CAD build for the part. Positions are in the model's coordinates, mm. A direction names the side the tool comes from. Give positions to 0.01 mm unless a question says otherwise; leave off trailing zeros. Write each loop counter-clockwise with the first axis right and the second up, starting at its lowest first coordinate (ties: lowest second). Pieces come first, ordered by that corner, then holes. Notation, with made-up numbers: (1, 19) - (13, 19) arc R30 cw to (13, 53) - close; hole circle Ø10 at (66.25, 86). An arc over 180 degrees is marked (long way). Answer as a JSON object with one key per item and string values.
from build123d import *

# Parameters (mm, degrees)
SKETCH_1_R          = 2.1
EXTRUDE_1_DEPTH     = 2
CUT_EXTRUDE_1_DEPTH = 94.621578709
CHAMFER_1_SIZE      = 2
SKETCH_4_R          = 1
CUT_EXTRUDE_2_DEPTH = 94.621578709
CHAMFER_2_SIZE      = 4
SKETCH_7_R          = 1.6
CUT_EXTRUDE_3_DEPTH = 94.621578709


with BuildPart() as part:
    # 草图1 → 凸台-拉伸1 (new, symmetric)
    with BuildSketch(Plane.XY):
        with BuildLine():
            Line((11, 0), (-11, 0))
            Line((-11, 0), (-11, -82))
            Line((-11, -82), (-31, -82))
            Line((-31, -82), (-31, 20))
            Line((-31, 20), (45, 20))
            Line((45, 20), (45, -33.306562209))
            ThreePointArc((45, -33.306562209), (42.507569164, -36.65839818), (38.580111783, -35.236394534))
            Line((38.580111783, -35.236394534), (34, -28.306562209))
            Line((34, -28.306562209), (22, -28.306562209))
            Line((22, -28.306562209), (17.419888217, -35.236394534))
            ThreePointArc((17.419888217, -35.236394534), (13.492430836, -36.65839818), (11, -33.306562209))
            Line((11, -33.306562209), (11, 0))
        make_face()
        with Locations((-21, 10)):
            Circle(SKETCH_1_R, mode=Mode.SUBTRACT)
        with Locations((35, 10)):
            Circle(SKETCH_1_R, mode=Mode.SUBTRACT)
        with Locations((14.5, -33.306562209)):
            Circle(SKETCH_1_R, mode=Mode.SUBTRACT)
        with Locations((41.5, -33.306562209)):
            Circle(SKETCH_1_R, mode=Mode.SUBTRACT)
        with Locations((-21, -72)):
            Circle(SKETCH_1_R, mode=Mode.SUBTRACT)
    extrude(amount=EXTRUDE_1_DEPTH, both=True)

    # 草图3 → 切除-拉伸1 (cut, through all)
    with BuildSketch(Plane.XY.offset(2)):
        Polygon((-16, 20), (-11, 15), (25, 15), (30, 20), align=None)
    extrude(amount=-CUT_EXTRUDE_1_DEPTH, mode=Mode.SUBTRACT)

    # 倒角1
    chamfer_1_edges = [part.edges().sort_by_distance(p)[0] for p in [
        (-23.1, 10, -2),
        (32.9, 10, -2),
        (-23.1, -72, -2),
    ]]
    chamfer(chamfer_1_edges, length=CHAMFER_1_SIZE)

    # 草图4 → 切除-拉伸2 (cut, through all)
    with BuildSketch(Plane.XY.offset(2)):
        with Locations((-11, -1)):
            Circle(SKETCH_4_R)
        with Locations((11, -1)):
            Circle(SKETCH_4_R)
    extrude(amount=-CUT_EXTRUDE_2_DEPTH, mode=Mode.SUBTRACT)

    # 倒角2
    chamfer_2_edges = [part.edges().sort_by_distance(p)[0] for p in [
        (-11, -82, 0),
        (-31, -82, 0),
        (45, 20, 0),
    ]]
    chamfer(chamfer_2_edges, length=CHAMFER_2_SIZE)

    # 草图7 → 切除-拉伸3 (cut, through all)
    with BuildSketch(Plane.XY.offset(2)):
        with Locations((-28.5, -48)):
            Circle(SKETCH_7_R)
        with Locations((-28.5, -58)):
            Circle(SKETCH_7_R)
        with Locations((-13.5, -48)):
            Circle(SKETCH_7_R)
        with Locations((-13.5, -58)):
            Circle(SKETCH_7_R)
    extrude(amount=-CUT_EXTRUDE_3_DEPTH, mode=Mode.SUBTRACT)


solid = part.part
(1) Probe L1, parallel to Y at x = -21, z = 1.3; L2, parallel to Y at x = -21.5, z = 0.9; L3, parallel to X at y = -10, z = 0.1. List the from-to ranges inside material, lowest first. Write a range as [from, to].
Answer key:
{"L1": "y = [-82, -74.1], [-69.9, 7.9], [12.1, 20]", "L2": "y = [-82, -74.04], [-69.96, 7.96], [12.04, 20]", "L3": "x = [-31, -11], [11, 45]"}
(2) Pull direction Y, two halves, no side cores. Call faces 1 (the face through (-15.1, -47.93, 0.03)), 2 (the face through (36.32, -31.82, 0.03)), 3 (the face through (35, 20, 0)): pulls with the +Y half, pulls with the -Y half, needs draft (parallel to the pull), parting line crosses it, or undercut.
Answer key:
{"face 1": "undercut", "face 2": "pulls with the -Y half", "face 3": "pulls with the +Y half"}
(3) Flat gauge pins, fed straight in: P1, Ø2.5, axis at x = -28.5, y = -58, coming from the +Z side; P2, Ø2, axis at y = -58, z = 0.5, coming from the +X side; P3, Ø1, axis at x = 4.5, z = 0.5, coming from the +Y side. Where does each tip first touch, or does it go through?
Answer key:
{"P1": "passes through", "P2": "stops at x = -11", "P3": "stops at y = 15"}
(4) 3-axis set-ups, long thin cutter, end or side, ignore diameter. For faces 4 (the face through (-29, -80, 0)), 5 (the face through (7, 15, 0)), 6 (the face through (43, 18, 0)), 7 (the face through (12, -1, 0)), 8 (the face through (28, -28.307, 0)): which of +Z, -Z, +X, -X, +Y, -Y reach the whole face in a straight line?
Answer key:
{"face 4": "+Z, -Z, -X, -Y", "face 5": "+Z, -Z, +Y", "face 6": "+Z, -Z, +X, +Y", "face 7": "+Z, -Z", "face 8": "+Z, -Z, -Y"}
(5) Saw through at A-A, the plane y = -26. Give the cut face in (x, z), and give its area (3 significant figures).
Answer key:
{"outline": "(-31, -2) - (-11, -2) - (-11, 2) - (-31, 2) - close; (11, -2) - (45, -2) - (45, 2) - (11, 2) - close", "area": "216 mm²"}
(6) Saw through at D-D, the plane y = -58. Give the cut face in (x, z), and give its area (3 significant figures).
Answer key:
{"outline": "(-31, -2) - (-30.1, -2) - (-30.1, 2) - (-31, 2) - close; (-26.9, -2) - (-15.1, -2) - (-15.1, 2) - (-26.9, 2) - close; (-11.9, -2) - (-11, -2) - (-11, 2) - (-11.9, 2) - close", "area": "54.4 mm²"}
(7) Saw through at B-B, the plane z = 0.65. State how many separate pieces and enclosed holes the cut face has, and give its area (3 significant figures).
Answer key:
{"separate pieces": "1", "enclosed holes": "9", "area": "3,920 mm²"}
(8) Saw through at C-C, the plane x = -28.5. Give the cut face in (y, z), and give its area (3 significant figures).
Answer key:
{"outline": "(-80.5, -2) - (-59.6, -2) - (-59.6, 2) - (-80.5, 2) - close; (-56.4, -2) - (-49.6, -2) - (-49.6, 2) - (-56.4, 2) - close; (-46.4, -2) - (20, -2) - (20, 2) - (-46.4, 2) - close", "area": "376 mm²"}
